The listing builds one solid part. Answer for the finished solid, in the listing's coordinates (mm). Face numbers are marked on the shaded views. A direction names the side the tool comes from. Coordinates: 2 decimals unless noted, no trailing zeros. Order: outer loops, then holes, each group sorted by start corner. A loop starts at its lowest first (then second) coordinate and runs counter-clockwise, first axis right, second up. Notation, with made-up numbers: (52.25, -24) -> (80.25, -24) arc R19 ccw to (80.25, 11) -> close; hole circle Ø10 at (-34.5, 21.5). An arc over 180 degrees is marked (long way). One line per question, with ' | ' between items.
from build123d import *

# Parameters (mm, degrees)
SKETCH1_W            = 66.675
SKETCH1_H            = 52.2732
BOSS_EXTRUDE1_DEPTH  = 1.27
BOSS_EXTRUDE3_DEPTH  = 4.7625
BOSS_EXTRUDE4_DEPTH  = 7.9375
CUT_EXTRUDE2_DEPTH   = 2.921
FILLET1_R            = 1.27
FILLET2_R            = 1.27
MIRROR1_START        = 20.16125
MIRROR1_DEPTH        = 7.0485
MIRROR1_START_2      = 27.20975
MIRROR1_2_DEPTH      = 2.921
MIRROR1_START_3      = -8
MIRROR1_3_DEPTH      = 12
SKETCH7_W            = 1.016
SKETCH7_H            = 1.905
BOSS_EXTRUDE5_DEPTH  = 66.675
SKETCH8_W            = 66.675
SKETCH8_H            = 0.6604
BOSS_EXTRUDE6_DEPTH  = 0.762
FILLET5_R            = 1.651
SKETCH10_W           = 9.525
SKETCH10_H           = 2.7178
CUT_EXTRUDE3_DEPTH   = 0.1016
SKETCH11_W           = 66.675
SKETCH11_H           = 1.2446
CUT_EXTRUDE4_DEPTH   = 0.1016
SKETCH12_W           = 107.616027614
SKETCH12_H           = 63.046095141
SKETCH12_W_2         = 66.167
SKETCH12_H_2         = 53.768388695
CUT_EXTRUDE5_DEPTH   = 46.918560191
FILLET6_R            = 4.7625
SKETCH13_W           = 0.8636
SKETCH13_H           = 0.6604
CUT_EXTRUDE6_DEPTH   = 74.315736052
BOSS_EXTRUDE8_DEPTH  = 66.167
FILLET7_R            = 0.508
BOSS_EXTRUDE9_DEPTH  = 66.167
SKETCH17_W           = 9.525
SKETCH17_H           = 1.1684
BOSS_EXTRUDE10_DEPTH = 1.27
SKETCH18_W           = 12.7
SKETCH18_H           = 4.7625
BOSS_EXTRUDE13_DEPTH = 0.508
FILLET8_R            = 0.3048


with BuildPart() as part:
    # Sketch1 → Boss-Extrude1 (new body)
    with BuildSketch(Plane(origin=(0, 0, 0), x_dir=(1, 0, 0), z_dir=(0, 1, 0))):
        Rectangle(SKETCH1_W, SKETCH1_H)
    extrude(amount=BOSS_EXTRUDE1_DEPTH)

    # Sketch4 → Boss-Extrude3 (add, symmetric)
    with BuildSketch(Plane(origin=(0, 0, 0), x_dir=(0, 0, -1), z_dir=(1, 0, 0))):
        Polygon((28.987783874, 1.055971868), (31.3309, 1.683807942), (31.3309, 2.794), (18.1991, 2.794), (18.1991, 1.27), (26.1366, 1.27), (26.1366, 1.524), (28.8544, 1.524), (28.8544, 1.055971868), align=None)
    extrude(amount=BOSS_EXTRUDE3_DEPTH, both=True)

    # Sketch5 → Boss-Extrude4 (add)
    with BuildSketch(Plane(origin=(0, 0, -5.8166), x_dir=(-1, 0, 0), z_dir=(0, 0, -1))):
        Polygon((21.43125, 1.27), (27.20975, 1.27), (27.20975, 2.413), (30.13075, 2.413), (30.13075, 3.937), (21.43125, 3.937), align=None)
    extrude(amount=-BOSS_EXTRUDE4_DEPTH)

    # Sketch6 → Cut-Extrude2 (cut)
    with BuildSketch(Plane.ZY.offset(30.13075)):
        Polygon((-5.8166, 2.413), (-3.2766, 2.413), (-5.8166, 3.093590949), align=None)
    extrude(amount=-CUT_EXTRUDE2_DEPTH, mode=Mode.SUBTRACT)

    # Fillet1
    fillet1_edges = [part.edges().sort_by_distance(p)[0] for p in [
        (-24.3205, 1.27, 2.1209),
        (-21.43125, 1.27, -1.84785),
        (-24.3205, 1.27, -5.8166),
    ]]
    fillet(fillet1_edges, radius=FILLET1_R)

    # Fillet2
    # the kernel refuses this fillet: 1.27 mm, written as the material it adds along each edge
    with BuildSketch(Plane(origin=(-4.7625, 1.27, -18.1991), x_dir=(-1, 0, 0), z_dir=(0, 0, -1))) as fillet2_piece_1:
        with BuildLine():
            CenterArc((FILLET2_R, FILLET2_R), FILLET2_R, 180, 90)
            Line((0, FILLET2_R), (-FILLET2_R * 0.02, FILLET2_R))
            Line((-FILLET2_R * 0.02, FILLET2_R), (-FILLET2_R * 0.02, -FILLET2_R * 0.02))
            Line((-FILLET2_R * 0.02, -FILLET2_R * 0.02), (FILLET2_R, -FILLET2_R * 0.02))
            Line((FILLET2_R, -FILLET2_R * 0.02), (FILLET2_R, 0))
        make_face()
    extrude(amount=7.9375)
    with BuildSketch(Plane(origin=(-4.7625, 1.27, -18.1991), x_dir=(0, 0, 1), z_dir=(1, 0, 0))) as fillet2_piece_2:
        with BuildLine():
            CenterArc((FILLET2_R, -FILLET2_R), FILLET2_R, 90, 90)
            Line((0, -FILLET2_R), (-FILLET2_R * 0.02, -FILLET2_R))
            Line((-FILLET2_R * 0.02, -FILLET2_R), (-FILLET2_R * 0.02, FILLET2_R * 0.02))
            Line((-FILLET2_R * 0.02, FILLET2_R * 0.02), (FILLET2_R, FILLET2_R * 0.02))
            Line((FILLET2_R, FILLET2_R * 0.02), (FILLET2_R, 0))
        make_face()
    extrude(amount=9.525)
    with BuildSketch(Plane(origin=(4.7625, 1.27, -18.1991), x_dir=(1, 0, 0), z_dir=(0, 0, -1))) as fillet2_piece_3:
        with BuildLine():
            CenterArc((FILLET2_R, -FILLET2_R), FILLET2_R, 90, 90)
            Line((0, -FILLET2_R), (-FILLET2_R * 0.02, -FILLET2_R))
            Line((-FILLET2_R * 0.02, -FILLET2_R), (-FILLET2_R * 0.02, FILLET2_R * 0.02))
            Line((-FILLET2_R * 0.02, FILLET2_R * 0.02), (FILLET2_R, FILLET2_R * 0.02))
            Line((FILLET2_R, FILLET2_R * 0.02), (FILLET2_R, 0))
        make_face()
    extrude(amount=7.9375)
    with BuildSketch(Plane(origin=(-4.7625, 1.27, -15.0241), x_dir=(-1, 0, 0), z_dir=(0, 0, -1))) as fillet2_piece_4a_section:
        with BuildLine():
            CenterArc((FILLET2_R, FILLET2_R), FILLET2_R, 180, 90)
            Line((0, FILLET2_R), (-FILLET2_R * 0.02, FILLET2_R))
            Line((-FILLET2_R * 0.02, FILLET2_R), (-FILLET2_R * 0.02, -FILLET2_R * 0.02))
            Line((-FILLET2_R * 0.02, -FILLET2_R * 0.02), (FILLET2_R, -FILLET2_R * 0.02))
            Line((FILLET2_R, -FILLET2_R * 0.02), (FILLET2_R, 0))
        make_face()
    fillet2_piece_4a = extrude(amount=11.1125, mode=Mode.PRIVATE)
    fillet2_piece_4a = split(fillet2_piece_4a, bisect_by=Plane(origin=(-4.7625, 1.27, -18.1991), z_dir=(0, 0, 1)), keep=Keep.TOP, mode=Mode.PRIVATE)
    with BuildSketch(Plane(origin=(-7.9375, 1.27, -18.1991), x_dir=(0, 0, 1), z_dir=(1, 0, 0))) as fillet2_piece_4b_section:
        with BuildLine():
            CenterArc((FILLET2_R, -FILLET2_R), FILLET2_R, 90, 90)
            Line((0, -FILLET2_R), (-FILLET2_R * 0.02, -FILLET2_R))
            Line((-FILLET2_R * 0.02, -FILLET2_R), (-FILLET2_R * 0.02, FILLET2_R * 0.02))
            Line((-FILLET2_R * 0.02, FILLET2_R * 0.02), (FILLET2_R, FILLET2_R * 0.02))
            Line((FILLET2_R, FILLET2_R * 0.02), (FILLET2_R, 0))
        make_face()
    fillet2_piece_4b = extrude(amount=12.7, mode=Mode.PRIVATE)
    fillet2_piece_4b = split(fillet2_piece_4b, bisect_by=Plane(origin=(-4.7625, 1.27, -18.1991), z_dir=(-1, 0, 0)), keep=Keep.TOP, mode=Mode.PRIVATE)
    fillet2_piece_4 = fillet2_piece_4a & fillet2_piece_4b
    add(fillet2_piece_4)
    with BuildSketch(Plane(origin=(-4.7625, 1.27, -18.1991), x_dir=(0, 0, 1), z_dir=(1, 0, 0))) as fillet2_piece_5a_section:
        with BuildLine():
            CenterArc((FILLET2_R, -FILLET2_R), FILLET2_R, 90, 90)
            Line((0, -FILLET2_R), (-FILLET2_R * 0.02, -FILLET2_R))
            Line((-FILLET2_R * 0.02, -FILLET2_R), (-FILLET2_R * 0.02, FILLET2_R * 0.02))
            Line((-FILLET2_R * 0.02, FILLET2_R * 0.02), (FILLET2_R, FILLET2_R * 0.02))
            Line((FILLET2_R, FILLET2_R * 0.02), (FILLET2_R, 0))
        make_face()
    fillet2_piece_5a = extrude(amount=12.7, mode=Mode.PRIVATE)
    fillet2_piece_5a = split(fillet2_piece_5a, bisect_by=Plane(origin=(4.7625, 1.27, -18.1991), z_dir=(1, 0, 0)), keep=Keep.TOP, mode=Mode.PRIVATE)
    with BuildSketch(Plane(origin=(4.7625, 1.27, -15.0241), x_dir=(1, 0, 0), z_dir=(0, 0, -1))) as fillet2_piece_5b_section:
        with BuildLine():
            CenterArc((FILLET2_R, -FILLET2_R), FILLET2_R, 90, 90)
            Line((0, -FILLET2_R), (-FILLET2_R * 0.02, -FILLET2_R))
            Line((-FILLET2_R * 0.02, -FILLET2_R), (-FILLET2_R * 0.02, FILLET2_R * 0.02))
            Line((-FILLET2_R * 0.02, FILLET2_R * 0.02), (FILLET2_R, FILLET2_R * 0.02))
            Line((FILLET2_R, FILLET2_R * 0.02), (FILLET2_R, 0))
        make_face()
    fillet2_piece_5b = extrude(amount=11.1125, mode=Mode.PRIVATE)
    fillet2_piece_5b = split(fillet2_piece_5b, bisect_by=Plane(origin=(4.7625, 1.27, -18.1991), z_dir=(0, 0, 1)), keep=Keep.TOP, mode=Mode.PRIVATE)
    fillet2_piece_5 = fillet2_piece_5a & fillet2_piece_5b
    add(fillet2_piece_5)

    # Mirror1: read off the stored shape, not the designer's step
    # Mirror1 outline → Mirror1 (add)
    with BuildSketch(Plane.YZ.offset(MIRROR1_START)):
        with BuildLine():
            Line((3.937, -5.8166), (3.937, 2.1209))
            Line((3.937, 2.1209), (2.54, 2.1209))
            ThreePointArc((2.54, 2.1209), (1.641974388, 2.492874388), (1.27, 3.3909))
            Line((1.27, 3.3909), (1.27, -7.0866))
            ThreePointArc((1.27, -7.0866), (1.641974388, -6.188574388), (2.54, -5.8166))
            Line((2.54, -5.8166), (3.937, -5.8166))
        make_face()
    extrude(amount=MIRROR1_DEPTH)

    # Mirror1 2 outline → Mirror1 2 (add)
    with BuildSketch(Plane.YZ.offset(MIRROR1_START_2)):
        with BuildLine():
            Line((3.937, -5.8166), (3.937, 2.1209))
            Line((3.937, 2.1209), (2.54, 2.1209))
            ThreePointArc((2.54, 2.1209), (2.476420276, 2.122492487), (2.413, 2.127265955))
            Line((2.413, 2.127265955), (2.413, -5.822965955))
            ThreePointArc((2.413, -5.822965955), (2.476420276, -5.818192487), (2.54, -5.8166))
            Line((2.54, -5.8166), (3.937, -5.8166))
        make_face()
    extrude(amount=MIRROR1_2_DEPTH)

    # Mirror1 3 outline → Mirror1 3 (cut)
    with BuildSketch(Plane.XY.offset(MIRROR1_START_3)):
        with BuildLine():
            ThreePointArc((20.16125, 1.27), (21.059275612, 1.641974388), (21.43125, 2.54))
            Line((21.43125, 2.54), (21.43125, 3.937))
            Line((21.43125, 3.937), (20.16125, 3.937))
            Line((20.16125, 3.937), (20.16125, 1.27))
        make_face()
    extrude(amount=MIRROR1_3_DEPTH, mode=Mode.SUBTRACT)

    # Sketch7 → Boss-Extrude5 (add)
    with BuildSketch(Plane.ZY.offset(33.3375)):
        with Locations((25.6286, 2.2225)):
            Rectangle(SKETCH7_W, SKETCH7_H)
    extrude(amount=-BOSS_EXTRUDE5_DEPTH)

    # Sketch8 → Boss-Extrude6 (add)
    with BuildSketch(Plane(origin=(0, 0, 25.1206), x_dir=(-1, 0, 0), z_dir=(0, 0, -1))):
        with Locations((0, 2.8448)):
            Rectangle(SKETCH8_W, SKETCH8_H)
    extrude(amount=BOSS_EXTRUDE6_DEPTH)

    # Fillet5
    fillet5_edges = [part.edges().sort_by_distance(p)[0] for p in [
        (0, 0, 26.1366),
    ]]
    fillet(fillet5_edges, radius=FILLET5_R)

    # Sketch10 → Cut-Extrude3 (cut)
    with BuildSketch(Plane.XZ.offset(-1.524)):
        with Locations((0, -27.4955)):
            Rectangle(SKETCH10_W, SKETCH10_H)
    extrude(amount=-CUT_EXTRUDE3_DEPTH, mode=Mode.SUBTRACT)

    # Sketch11 → Cut-Extrude4 (cut)
    with BuildSketch(Plane(origin=(0, 0, 25.1206), x_dir=(-1, 0, 0), z_dir=(0, 0, -1))):
        with Locations((0, 1.8923)):
            Rectangle(SKETCH11_W, SKETCH11_H)
    extrude(amount=-CUT_EXTRUDE4_DEPTH, mode=Mode.SUBTRACT)

    # Sketch12 → Cut-Extrude5 (cut, through all)
    with BuildSketch(Plane.XZ):
        with Locations((0, 4.37044757)):
            Rectangle(SKETCH12_W, SKETCH12_H)
        with Locations((0, 1.001594348)):
            Rectangle(SKETCH12_W_2, SKETCH12_H_2, mode=Mode.SUBTRACT)
    extrude(amount=-CUT_EXTRUDE5_DEPTH, mode=Mode.SUBTRACT)


with BuildPart() as cut_extrude5_piece_1:
    # of the separate pieces the step leaves, piece 1, a body of its own (cut_extrude5_pieces)
    add(part.part.solids().sort_by_distance((33.0835, 1.651, 26.1366))[0])

    # Fillet6
    fillet6_edges = [cut_extrude5_piece_1.edges().sort_by_distance(p)[0] for p in [
        (-33.0835, 0.635, -25.8826),
        (33.0835, 0.635, -25.8826),
    ]]
    fillet(fillet6_edges, radius=FILLET6_R)

    # Sketch13 → Cut-Extrude6 (cut, through all)
    with BuildSketch(Plane.ZY.offset(33.0835)):
        with Locations((24.7904, 2.8448)):
            Rectangle(SKETCH13_W, SKETCH13_H)
    extrude(amount=-CUT_EXTRUDE6_DEPTH, mode=Mode.SUBTRACT)

    # Sketch14 → Boss-Extrude8 (add)
    with BuildSketch(Plane.ZY.offset(33.0835)):
        Polygon((25.2222, 3.175), (24.5872, 3.175), (24.5872, 2.54), (25.2222, 1.905), align=None)
    extrude(amount=-BOSS_EXTRUDE8_DEPTH)

    # Fillet7
    fillet7_edges = [cut_extrude5_piece_1.edges().sort_by_distance(p)[0] for p in [
        (0, 1.27, 25.2222),
    ]]
    fillet(fillet7_edges, radius=FILLET7_R)

    # Sketch16 → Boss-Extrude9 (add)
    with BuildSketch(Plane.ZY.offset(33.0835)):
        Polygon((25.2222, 3.175), (24.4602, 3.175), (24.4602, 2.6162), (25.2222, 1.8542), align=None)
    extrude(amount=-BOSS_EXTRUDE9_DEPTH)



with BuildPart() as cut_extrude5_piece_2:
    # of the separate pieces the step leaves, piece 2, a body of its own (cut_extrude5_pieces)
    add(part.part.solids().sort_by_distance((4.7625, 1.6256, -27.1526))[0])


with BuildPart() as cut_extrude5_piece_1_1:
    add(cut_extrude5_piece_1.part)

    add(cut_extrude5_piece_2.part)  # Boss-Extrude10 merges Cut-Extrude5 piece 2
    # Sketch17 → Boss-Extrude10 (add)
    with BuildSketch(Plane.XY.offset(-27.1526)):
        with Locations((0, 2.2098)):
            Rectangle(SKETCH17_W, SKETCH17_H)
    extrude(amount=BOSS_EXTRUDE10_DEPTH)

    # Sketch18 → Boss-Extrude13 (add)
    with BuildSketch(Plane.XZ):
        with Locations((0, -20.32635)):
            Rectangle(SKETCH18_W, SKETCH18_H)
    extrude(amount=BOSS_EXTRUDE13_DEPTH)

    # Fillet8
    fillet8_edges = [cut_extrude5_piece_1_1.edges().sort_by_distance(p)[0] for p in [
        (6.35, -0.254, -22.7076),
        (6.35, -0.254, -17.9451),
        (-6.35, -0.254, -17.9451),
        (-6.35, -0.254, -22.7076),
        (6.35, -0.508, -20.32635),
        (0, -0.508, -17.9451),
        (-6.35, -0.508, -20.32635),
        (0, -0.508, -22.7076),
    ]]
    fillet(fillet8_edges, radius=FILLET8_R)


solid = cut_extrude5_piece_1_1.part
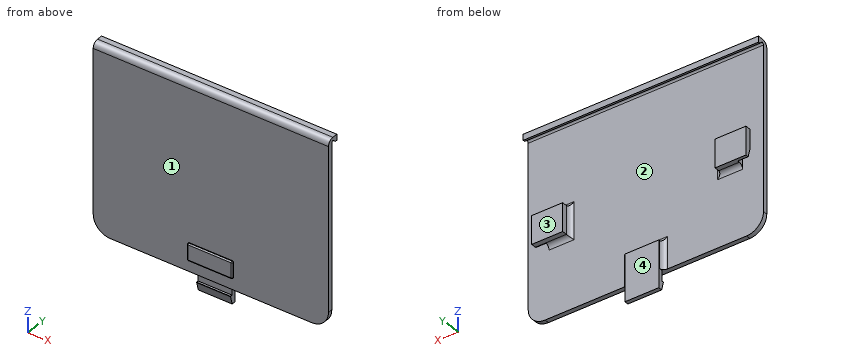
Item 1: Each of these flat-tipped pins is pushed along its axis until it touches: pin 1 Ø5 at (x, z) = (-1.5, -27) entering from +Y; pin 2 Ø12 at (x, z) = (24.5, 15) entering from +Y; pin 3 Ø0.9 at (y, z) = (2, -2) entering from -X; pin 4 Ø1.1 at (x, y) = (27, 3.5) entering from +Z. Where does it stop, or does it pass through?
Computed values:
pin 1: stops at y = 2.79 | pin 2: stops at y = 1.27 | pin 3: stops at x = -30.13 | pin 4: stops at z = 26.14
Item 2: Section B-B, the plane z = -2.5 is taken. Give the vertices of the cut face in (x, y), plus the area to 3 significant figures.
Computed values:
outline: (-33.08, 0) -> (33.08, 0) -> (33.08, 1.27) -> (27.21, 1.27) -> (27.21, 2.41) -> (30.13, 2.41) -> (30.13, 3.94) -> (21.43, 3.94) -> (21.43, 2.54) arc R1.27 cw to (20.16, 1.27) -> (-20.16, 1.27) arc R1.27 cw to (-21.43, 2.54) -> (-21.43, 3.94) -> (-30.13, 3.94) -> (-30.13, 2.41) -> (-27.21, 2.41) -> (-27.21, 1.27) -> (-33.08, 1.27) -> close | area: 124 mm^2
Item 3: Determine the mould class of the marked faces 1 and 2 for opening direction Z: pulls with the +Z half, pulls with the -Z half, needs draft (parallel to the pull), parting line crosses it, or undercut.
Computed values:
face 1: needs draft | face 2: undercut
Item 4: Section A-A, the plane x = 9 is taken. Give the vertices of the cut face in (y, z) (3 decimals), plus the area to 3 significant figures.
Computed values:
outline: (0, -25.883) -> (1.27, -25.883) -> (1.27, 24.714) arc R0.508 cw to (1.778, 25.222) -> (1.854, 25.222) -> (2.616, 24.46) -> (3.175, 24.46) -> (3.175, 26.137) -> (1.651, 26.137) arc R1.651 ccw to (0, 24.486) -> close | area: 68.0 mm^2
Item 5: For the marked faces 3 and 4, determine the directions among +Z, -Z, +X, -X, +Y, -Y from which every point of the face is accessible in a straight line to the end or side of a thin tool.
Computed values:
face 3: +Z, -Z, +X, -X, +Y | face 4: -Z, +X, -X, +Y
Item 6: Section C-C, the plane x = 26 is taken. Give the vertices of the cut face in (y, z) (3 decimals), plus the area to 3 significant figures.
Computed values:
outline: (0, -25.883) -> (1.27, -25.883) -> (1.27, -7.087) arc R1.27 cw to (2.54, -5.817) -> (3.937, -5.817) -> (3.937, 2.121) -> (2.54, 2.121) arc R1.27 cw to (1.27, 3.391) -> (1.27, 24.714) arc R0.508 cw to (1.778, 25.222) -> (1.854, 25.222) -> (2.616, 24.46) -> (3.175, 24.46) -> (3.175, 26.137) -> (1.651, 26.137) arc R1.651 ccw to (0, 24.486) -> close | area: 89.9 mm^2
Item 7: Section D-D, the plane z = 15.5 is taken. Give the vertices of the cut face in (x, y), plus the area to 3 significant figures.
Computed values:
outline: (-33.08, 0) -> (33.08, 0) -> (33.08, 1.27) -> (-33.08, 1.27) -> close | area: 84.0 mm^2
Item 8: Find the intervals of material crossed by L1, parallel to Y at x = 15, z = 2.5; L2, parallel to Z at x = -25, y = 1.7; L3, parallel to Z at x = -11, y = 2.75, in increasing order.
Computed values:
L1: y = 0 to 1.27 | L2: z = -6.13 to 2.44, 25.22 to 26.14 | L3: z = 24.46 to 26.14
